For this review, take the finished solid that the model builds, in its own axes (mm). Face numbers are marked on the shaded views. A direction names the side the tool comes from. Give positions to 0.01 mm unless a question says otherwise; leave off trailing zeros. Write each loop counter-clockwise with the first axis right and the second up, starting at its lowest first coordinate (ties: lowest second). Pieces come first, ordered by that corner, then holes. Notation, with made-up numbers: M 22,-4.5 L 37,-4.5 A28 cw 37,31.5 Z; hole C 82,-13 d11. An arc over 180 degrees is marked long. Write item = value, one per line.
```python
from build123d import *

# Parameters (mm, degrees)
F1_DEPTH = 5.3


with BuildPart() as f1:
    # F0 (on Top) → F1 (new body)
    with BuildSketch(Plane.XY):
        Polygon((36.987744, -22.647183), (0, 37.559837), (-32.954307, -22.647183), align=None)
        Polygon((31.247444, -19.210724), (0, -19.210724), (-28.124915, -19.210724), (0, 32.173071), align=None, mode=Mode.SUBTRACT)
    extrude(amount=F1_DEPTH)


solid = f1.part
```
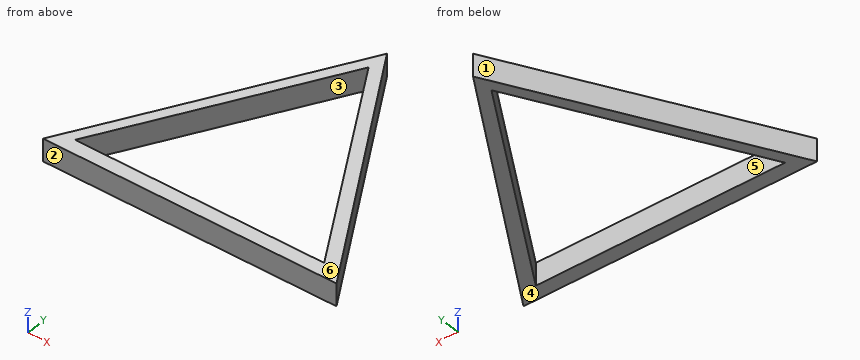
1. We need section B-B, the plane y = -2.5. Write out the cut boundary in (x, z), then the cut area to 3 significant figures.
Responses:
outline = M -21.93,0 L -18.98,0 L -18.98,5.3 L -21.93,5.3 Z; M 21.09,0 L 24.61,0 L 24.61,5.3 L 21.09,5.3 Z
area = 34.3 mm2
2. Machinability: for the marked faces 5 and 6, which of the approach directions +Z, -Z, +X, -X, +Y, -Y give a long, thin tool a straight path to every point of the face, cutting with its end or side? Answer none if there is none.
Responses:
face_5 = +Z, -Z
face_6 = +Z, +X, -X, +Y, -Y
3. Insertion check: P1, Ø1.6, axis at x = -1.5, z = 3, coming from the +Y side; P2, Ø3, axis at y = -16, z = 3.5, coming from the -X side; P3, Ø3, axis at x = 25.5, z = 4.5, coming from the +Y side. Each pin has a flat end and moves straight along its axis. Give the tip position at first contact, or say it passes through.
Responses:
P1 = 36.28
P2 = -30.14
P3 = -1.51
4. We need section A-A, the plane z = 1.35. Write out the cut boundary in (x, y), then the cut area to 3 significant figures.
Responses:
outline = M -32.95,-22.65 L 36.99,-22.65 L 0,37.56 Z; hole M -28.12,-19.21 L 31.25,-19.21 L 0,32.17 Z
area = 580 mm2
5. For line 1 along X through (y, z) = (4.5, 0.25); line 2 along Y through (x, z) = (-12, 4.5); line 3 along Y through (x, z) = (20.5, 3.75), list the stretches that pass through material, from the lowest coordinate up. Write a range as from..to.
Responses:
line_1 = -18.1..-15.15, 16.83..20.31
line_2 = -22.65..-19.21, 10.25..15.64
line_3 = -22.65..-19.21, -1.54..4.19
6. The part is to be moulded in two halves that separate along Y. For the marked faces 1, 2, 3 and 4, say which applies: +Y half, -Y half, draft (parallel to the pull), parting line (faces both ways), or undercut.
Responses:
face_1 = +Y half
face_2 = -Y half
face_3 = undercut
face_4 = draft
7. We need section C-C, the plane x = 22. Write out the cut boundary in (y, z), then the cut area to 3 significant figures.
Responses:
outline = M -22.65,0 L -19.21,0 L -19.21,5.3 L -22.65,5.3 Z; M -4,0 L 1.75,0 L 1.75,5.3 L -4,5.3 Z
area = 48.7 mm2
8. We need section D-D, the plane y = 33. Write out the cut boundary in (x, z), then the cut area to 3 significant figures.
Responses:
outline = M -2.5,0 L 2.8,0 L 2.8,5.3 L -2.5,5.3 Z
area = 28.1 mm2
